The listing builds one solid part. Answer for the finished solid, in the listing's coordinates (mm). Give positions to 0.01 mm unless a question says otherwise; leave off trailing zeros. Write each loop counter-clockwise with the first axis right and the second up, starting at its lowest first coordinate (ties: lowest second). Pieces come first, ordered by that corner, then holes. Notation, with made-up numbers: (-31, 18) - (-3, 18) arc R19 cw to (-3, 29) - close; hole circle Ø1 at (-3, 74). An arc over 180 degrees is marked (long way). Answer as CSV lines item,"result". Start each with the question number.
(1) Find section B-B (z = -5.5). Write down the section's boundary in (x, y), then the cut area to 3 significant figures.
(2) Find section A-A (x = 32). State how many separate pieces and enclosed holes the cut face has, then the cut area to 3 significant figures.
(3) Straight lines are drawn through the part: probe 1 along X at (y, z) = (206, 18.5); probe 2 along Y at (x, z) = (18, -87); probe 3 along Z at (x, y) = (57.5, 219.5). For each, find the intervals that lie inside material, in ascending order.
(4) Each of these flat-tipped pins is pushed along its axis until it touches: pin 1 Ø8 at (x, y) = (289.5, 56) entering from +Z; pin 2 Ø3 at (x, y) = (63.5, 132.5) entering from -Z; pin 3 Ø5.5 at (x, y) = (119.5, 5.5) entering from -Z. Where does it stop, or does it pass through?
from build123d import *

# Parameters (mm, degrees)
SKETCH1_W           = 406.4
SKETCH1_H           = 254
SKETCH1_W_2         = 368.3
SKETCH1_H_2         = 215.9
BOSS_EXTRUDE1_DEPTH = 25.4
SKETCH2_R           = 12.7
BOSS_EXTRUDE2_DEPTH = 368.3
SKETCH3_W           = 19.05
SKETCH3_H           = 19.05
BOSS_EXTRUDE3_DEPTH = 127


with BuildPart() as part:
    # Sketch1 → Boss-Extrude1 (new body)
    with BuildSketch(Plane.XY):
        with Locations((203.2, 127)):
            Rectangle(SKETCH1_W, SKETCH1_H)
        with Locations((203.2, 127)):
            Rectangle(SKETCH1_W_2, SKETCH1_H_2, mode=Mode.SUBTRACT)
    extrude(amount=BOSS_EXTRUDE1_DEPTH)

    # Sketch2 → Boss-Extrude2 (add)
    with BuildSketch(Plane(origin=(19.05, 0, 0), x_dir=(0, 0, -1), z_dir=(1, 0, 0))):
        with Locations(Location((-13.001554518, 219.046700044, 0), (0, 0, 192.51070534))):
            Circle(SKETCH2_R)
        with Locations(Location((-13.001554518, 188.566700044, 0), (0, 0, 192.51070534))):
            Circle(SKETCH2_R)
        with Locations(Location((-13.001554518, 158.086700044, 0), (0, 0, 192.51070534))):
            Circle(SKETCH2_R)
        with Locations(Location((-13.001554518, 127.606700044, 0), (0, 0, 192.51070534))):
            Circle(SKETCH2_R)
        with Locations(Location((-13.001554518, 97.126700044, 0), (0, 0, 192.51070534))):
            Circle(SKETCH2_R)
        with Locations(Location((-13.001554518, 66.646700044, 0), (0, 0, 192.51070534))):
            Circle(SKETCH2_R)
        with Locations(Location((-13.001554518, 36.166700044, 0), (0, 0, 192.51070534))):
            Circle(SKETCH2_R)
    extrude(amount=BOSS_EXTRUDE2_DEPTH)

    # Sketch3 → Boss-Extrude3 (add)
    with BuildSketch(Plane(origin=(0, 0, 0), x_dir=(-1, 0, 0), z_dir=(0, 0, -1))):
        with Locations((-396.875, 244.475)):
            Rectangle(SKETCH3_W, SKETCH3_H)
        with Locations((-396.875, 9.525)):
            Rectangle(SKETCH3_W, SKETCH3_H)
        with Locations((-9.525, 244.475)):
            Rectangle(SKETCH3_W, SKETCH3_H)
        with Locations((-9.525, 9.525)):
            Rectangle(SKETCH3_W, SKETCH3_H)
    extrude(amount=BOSS_EXTRUDE3_DEPTH)


solid = part.part
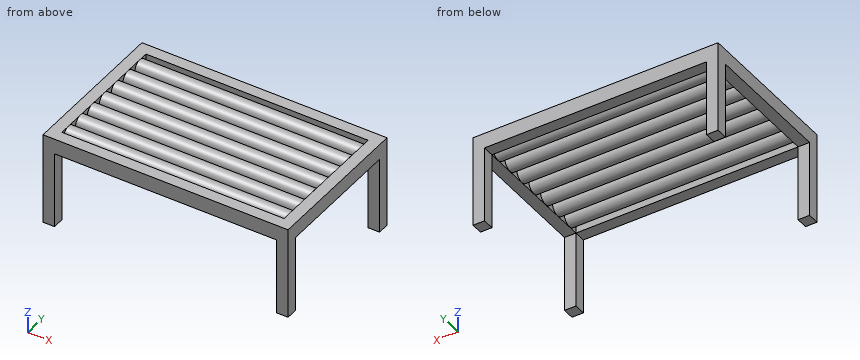
Result set:
1,outline,"(0, 0) - (19.05, 0) - (19.05, 19.05) - (0, 19.05) - close; (0, 234.95) - (19.05, 234.95) - (19.05, 254) - (0, 254) - close; (387.35, 0) - (406.4, 0) - (406.4, 19.05) - (387.35, 19.05) - close; (387.35, 234.95) - (406.4, 234.95) - (406.4, 254) - (387.35, 254) - close"
1,area,"1,450 mm^2"
2,separate pieces,"9"
2,enclosed holes,"0"
2,area,"4,510 mm^2"
3,probe 1,"0 to 19.05, 387.35 to 406.4"
3,probe 2,"0 to 19.05, 234.95 to 254"
3,probe 3,"0.31 to 25.69"
4,pin 1,"z = 23.82"
4,pin 2,"z = 0.76"
4,pin 3,"z = 0"
